The listing builds one solid part. Answer for the finished solid, in the listing's coordinates (mm). Face numbers are marked on the shaded views. A direction names the side the tool comes from. Round coordinates to 2 decimals unless told otherwise and drop trailing zeros. Write each loop counter-clockwise with the first axis right and the second up, starting at its lowest first coordinate (ties: lowest second). Pieces come first, ordered by that corner, then holes.
from build123d import *
from build123d.topology import SkipClean

# Parameters (mm, degrees)
SKETCH1_R               = 11
SKETCH1_R_2             = 4
BOSS_EXTRUDE1_DEPTH     = 10
SKETCH3_R               = 15.556349186
SKETCH3_R_2             = 11
BOSS_EXTRUDE2_DEPTH     = 4
CUT_EXTRUDE1_DEPTH      = 33.68393631
CUT_EXTRUDE1_DEPTH_BACK = 5.6
BOSS_EXTRUDE4_DEPTH     = 10
BOSS_EXTRUDE3_DEPTH     = 8
BOSS_EXTRUDE5_START     = 4
SKETCH3_2_R             = 15.556349186
SKETCH3_2_R_2           = 11
BOSS_EXTRUDE5_DEPTH     = 2
CUT_EXTRUDE2_DEPTH      = 37.349590584
CUT_EXTRUDE2_DEPTH_BACK = 5.6
CUT_EXTRUDE3_DEPTH      = 47.993816701
CUT_EXTRUDE3_DEPTH_BACK = 47.993816701
SKETCH13_R              = 7
CUT_EXTRUDE5_DEPTH      = 52.642447787
CUT_EXTRUDE5_DEPTH_BACK = 52.642447787
SKETCH14_R              = 1.5
SKETCH15_R              = 11.789942891
CUT_EXTRUDE6_DEPTH      = 8
BOSS_EXTRUDE6_REACH     = 48.308
SKETCH16_R              = 2


with BuildPart() as part:
    # Sketch1 → Boss-Extrude1 (new body)
    with BuildSketch(Plane(origin=(0, 0, 0), x_dir=(1, 0, 0), z_dir=(0, 1, 0))):
        with Locations(Location((0, 0, 0), (0, 0, 270))):
            Circle(SKETCH1_R)
        with Locations(Location((0, 0, 0), (0, 0, 270))):
            Circle(SKETCH1_R_2, mode=Mode.SUBTRACT)
    extrude(amount=BOSS_EXTRUDE1_DEPTH)

    # Sketch3 → Boss-Extrude2 (add, symmetric)
    with BuildSketch(Plane(origin=(0, 0, 0), x_dir=(0, 0, -1), z_dir=(1, 0, 0))):
        with Locations((0, 21)):
            Circle(SKETCH3_R)
        with Locations(Location((0, 21, 0), (0, 0, 270))):
            Circle(SKETCH3_R_2, mode=Mode.SUBTRACT)
    extrude(amount=BOSS_EXTRUDE2_DEPTH, both=True)

    # Sketch2 → Cut-Extrude1 (cut, two sides: drawn at the far end of the back side and taken through both)
    with BuildSketch(Plane(origin=(0, 10, 0), x_dir=(1, 0, 0), z_dir=(0, 1, 0)).offset(-CUT_EXTRUDE1_DEPTH_BACK)):
        Polygon((3.983716857, 6.9), (-3.983716857, 6.9), (-7.967433715, 0), (-3.983716857, -6.9), (3.983716857, -6.9), (7.967433715, 0), align=None)
    extrude(amount=CUT_EXTRUDE1_DEPTH + CUT_EXTRUDE1_DEPTH_BACK, mode=Mode.SUBTRACT)

    # Sketch9 → Boss-Extrude4 (add)
    with BuildSketch(Plane(origin=(0, 10, 0), x_dir=(1, 0, 0), z_dir=(0, 1, 0))):
        with BuildLine():
            ThreePointArc((4, -10.246950766), (11, 0), (4, 10.246950766))
            Line((4, 10.246950766), (4, 6.87179677))
            Line((4, 6.87179677), (7.967433715, 0))
            Line((7.967433715, 0), (4, -6.87179677))
            Line((4, -6.87179677), (4, -10.246950766))
        make_face()
    extrude(amount=BOSS_EXTRUDE4_DEPTH)

    # Sketch4 → Boss-Extrude3 (add)
    with BuildSketch(Plane(origin=(4, 0, 0), x_dir=(0, 0, -1), z_dir=(1, 0, 0))):
        with BuildLine():
            Line((-6.87179677, 34.956303563), (-6.87179677, 40.956303563))
            Line((-6.87179677, 40.956303563), (-13.914375327, 40.956303563))
            Line((-13.914375327, 40.956303563), (-13.914375327, 27.956303563))
            ThreePointArc((-13.914375327, 27.956303563), (-10.966596446, 32.033302425), (-6.87179677, 34.956303563))
        make_face()
        with BuildLine():
            Line((6.87179677, 34.956303563), (6.87179677, 40.956303563))
            Line((6.87179677, 40.956303563), (13.914375327, 40.956303563))
            Line((13.914375327, 40.956303563), (13.914375327, 27.956303563))
            ThreePointArc((13.914375327, 27.956303563), (10.966596446, 32.033302425), (6.87179677, 34.956303563))
        make_face()
    extrude(amount=-BOSS_EXTRUDE3_DEPTH)

    # Sketch3<2> → Boss-Extrude5 (add)
    # profile 1 of 2: a face of its own
    with SkipClean():  # the faces are left unmerged after this step: merging them gives an invalid solid
        with BuildSketch(Plane(origin=(0, 0, 0), x_dir=(0, 0, -1), z_dir=(1, 0, 0)).offset(BOSS_EXTRUDE5_START)):
            with Locations((0, 21)):
                Circle(SKETCH3_2_R)
            with Locations((0, 21)):
                Circle(SKETCH3_2_R_2, mode=Mode.SUBTRACT)
        # profile 2 of 2: a face of its own
        with BuildSketch(Plane(origin=(0, 0, 0), x_dir=(0, 0, -1), z_dir=(1, 0, 0)).offset(BOSS_EXTRUDE5_START)):
            with Locations((0, 21)):
                Circle(SKETCH3_2_R_2)
        extrude(amount=BOSS_EXTRUDE5_DEPTH)
    add(part.part.scale(1), mode=Mode.REPLACE)  # the faces are merged on a copy

    # Sketch2<2> → Cut-Extrude2 (cut, two sides: drawn at the far end of the back side and taken through both)
    with BuildSketch(Plane(origin=(0, 10, 0), x_dir=(1, 0, 0), z_dir=(0, 1, 0)).offset(-CUT_EXTRUDE2_DEPTH_BACK)):
        Polygon((3.983716857, 6.9), (-3.983716857, 6.9), (-7.967433715, 0), (-3.983716857, -6.9), (3.983716857, -6.9), (7.967433715, 0), align=None)
    extrude(amount=CUT_EXTRUDE2_DEPTH + CUT_EXTRUDE2_DEPTH_BACK, mode=Mode.SUBTRACT)

    # Sketch13 → Cut-Extrude3 (cut, two sides: drawn at the far end of the back side and taken through both)
    with BuildSketch(Plane(origin=(6, 0, 0), x_dir=(0, 0, -1), z_dir=(1, 0, 0)).offset(-CUT_EXTRUDE3_DEPTH_BACK)):
        with Locations((0, 21)):
            Circle(SKETCH13_R)
    extrude(amount=CUT_EXTRUDE3_DEPTH + CUT_EXTRUDE3_DEPTH_BACK, mode=Mode.SUBTRACT)

    # Sketch14 → Cut-Extrude5 (cut, two sides: drawn at the far end of the back side and taken through both)
    with BuildSketch(Plane.XY.offset(13.914375327).offset(-CUT_EXTRUDE5_DEPTH_BACK)):
        with Locations((0, 36.956303563)):
            Circle(SKETCH14_R)
        with BuildLine():
            Line((-4, 36.956303563), (-4, 43.473651887))
            Line((-4, 43.473651887), (4, 43.473651887))
            Line((4, 43.473651887), (4, 36.956303563))
            ThreePointArc((4, 36.956303563), (0, 40.956303563), (-4, 36.956303563))
        make_face()
    extrude(amount=CUT_EXTRUDE5_DEPTH + CUT_EXTRUDE5_DEPTH_BACK, mode=Mode.SUBTRACT)

    # Sketch15 → Cut-Extrude6 (cut)
    with BuildSketch(Plane(origin=(6, 0, 0), x_dir=(0, 0, -1), z_dir=(1, 0, 0))):
        with Locations((0, 21)):
            Circle(SKETCH15_R)
    extrude(amount=CUT_EXTRUDE6_DEPTH, mode=Mode.SUBTRACT)

    # Boss-Extrude6: up to this face of the body (flat: up to its plane)
    boss_extrude6_end = Plane(part.part.faces().sort_by_distance((6, 22.369931635, -9.227258585))[0])
    # Sketch16 → Boss-Extrude6 (add, up to the picked face)
    with BuildSketch(Plane.ZY.offset(4), mode=Mode.PRIVATE) as boss_extrude6_sk1:
        with BuildLine():
            Line((13.723567505, 13.674449171), (25.599337953, 20.043155389))
            ThreePointArc((25.599337953, 20.043155389), (28.089469493, 26.975176866), (21.451586712, 30.167697662))
            Line((21.451586712, 30.167697662), (13.914375327, 27.956303563))
            ThreePointArc((13.914375327, 27.956303563), (15.554961016, 20.792183273), (13.723567505, 13.674449171))
        make_face()
        with Locations((23, 24.890158814)):
            Circle(SKETCH16_R, mode=Mode.SUBTRACT)
    boss_extrude6_tool1 = split(extrude(boss_extrude6_sk1.sketch, amount=-BOSS_EXTRUDE6_REACH, mode=Mode.PRIVATE), bisect_by=boss_extrude6_end, keep=Keep.BOTH, mode=Mode.PRIVATE)
    add(boss_extrude6_tool1.solids().sort_by(Axis((-4, 23.412763, 20.74002), (1, 0, 0)))[0])


solid = part.part
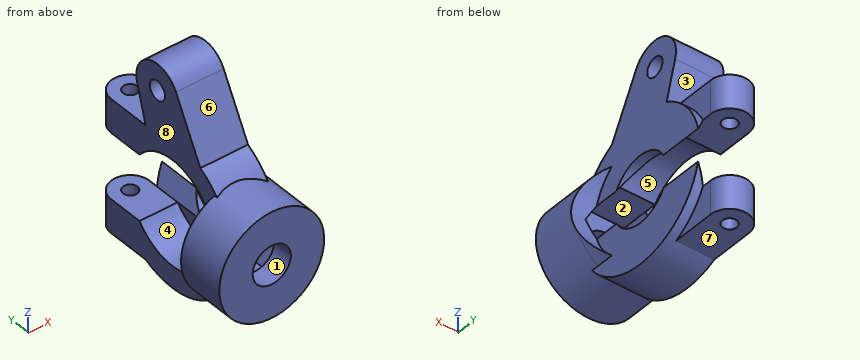
1. Straight lines are drawn through the part: line 1 along Z through (x, y) = (0.75, 26.5); line 2 along Y through (x, z) = (0, 8.75); line 3 along Y through (x, z) = (0.5, -9). For each, find the intervals that lie inside material, in ascending order.
Geometry says:
line 1: z = -14.55 to -9.53, 9.53 to 21.81, 24.19 to 28.26
line 2: y = 0 to 14.33, 27.67 to 35.46, 38.46 to 40.96
line 3: y = 0 to 14.68, 27.32 to 35.54, 38.37 to 40.92
2. For a pull along Z with two mould halves and no side action, classify the marked faces 5, 6, 7 and 8 as released by +Z, released by -Z, zero draft, split by the parting line, or undercut.
Geometry says:
face 5: undercut
face 6: released by +Z
face 7: released by -Z
face 8: zero draft
3. Given pin 1 (12 mm diameter, centred on x = 5, y = 4.5, fed in from +Z); pin 2 (2.5 mm diameter, centred on x = -2, y = 31.5, fed in from -Z); pin 3 (7.5 mm diameter, centred on y = 33, z = -9.5, fed in from +X), each flat-ended and moving along its own axis, determine where each tip first touches the part or whether it passes through.
Geometry says:
pin 1: stops at z = 11.48
pin 2: stops at z = -13.91
pin 3: stops at x = 6
4. Section A-A on x = 0 is taken. Give the number of separate pieces and of enclosed holes in the cut face, plus the area to 3 significant figures.
Geometry says:
separate pieces: 4
enclosed holes: 1
area: 561 mm2
5. Section B-B on y = 18.5 is taken. Determine the outline of the cut face in (x, z).
Geometry says:
outline: (-4, -15.35) - (6, -15.35) - (6, -6.54) - (4.19, -6.54) - (4, -6.87) - (4, -10.71) - (-4, -10.71) - close; (-4, 10.71) - (4, 10.71) - (4, 6.87) - (4.19, 6.54) - (6, 6.54) - (6, 22.72) - (-4, 22.72) - close
6. Section D-D on z = -8 is taken. Determine the outline of the cut face in (x, y), plus the area to 3 significant figures.
Geometry says:
outline: (-7.55, 0) - (7.55, 0) - (7.55, 12.34) - (6, 12.34) - (6, 34.34) - (4, 34.34) - (4, 36.96) arc R4 ccw to (-4, 36.96) - (-4, 28.55) - (4, 28.55) - (4, 13.45) - (-4, 13.45) - (-4, 10) - (-7.55, 10) - close; hole circle Ø3 at (0, 36.96)
area: 316 mm2
7. Section C-C on z = 23 is taken. Determine the outline of the cut face in (x, y).
Geometry says:
outline: (-4, 18.65) - (6, 18.65) - (6, 22.89) - (-4, 22.89) - close; (-4, 26.89) - (6, 26.89) - (6, 30.39) - (-4, 30.39) - close
8. A tool of negligible diameter and unlimited length cuts with its end or side. For the marked faces 1, 2, 3 and 4, from which of +Z, -Z, +X, -X, +Y, -Y can it reach the whole face along a straight path? Write none if from no direction.
Geometry says:
face 1: +Y, -Y
face 2: +Y
face 3: +X, -X, +Y
face 4: -X
